Source: CAD feature listing. Evaluate the final solid. Frame: model axes, mm. A direction names the side the tool comes from. Give positions to 0.01 mm unless a question says otherwise; leave off trailing zeros. Order: outer loops, then holes, each group sorted by start corner. A loop starts at its lowest first (then second) coordinate and runs counter-clockwise, first axis right, second up.
```python
from build123d import *

# Parameters (mm, degrees)
SKETCH_1_R          = 31
EXTRUDE_1_DEPTH     = 1
SKETCH_2_R          = 28.27
EXTRUDE_2_DEPTH     = 11
SKETCH_3_R          = 31
EXTRUDE_3_DEPTH     = 1
SKETCH_4_R          = 19
EXTRUDE_4_DEPTH     = 8
SKETCH_5_R          = 4
CUT_EXTRUDE_1_DEPTH = 49.610698411


with BuildPart() as part:
    # Эскиз1 → Бобышка-Вытянуть1 (new body)
    with BuildSketch(Plane(origin=(0, 0, 0), x_dir=(1, 0, 0), z_dir=(0, 1, 0))):
        with Locations(Location((0, 0, 0), (0, 0, 270))):
            Circle(SKETCH_1_R)
    extrude(amount=EXTRUDE_1_DEPTH)

    # Эскиз2 → Бобышка-Вытянуть2 (add)
    with BuildSketch(Plane(origin=(0, 1, 0), x_dir=(1, 0, 0), z_dir=(0, 1, 0))):
        with Locations(Location((0, 0, 0), (0, 0, 270))):
            Circle(SKETCH_2_R)
    extrude(amount=EXTRUDE_2_DEPTH)

    # Эскиз3 → Бобышка-Вытянуть3 (add)
    with BuildSketch(Plane(origin=(0, 12, 0), x_dir=(1, 0, 0), z_dir=(0, 1, 0))):
        with Locations(Location((0, 0, 0), (0, 0, 270))):
            Circle(SKETCH_3_R)
    extrude(amount=EXTRUDE_3_DEPTH)

    # Эскиз4 → Бобышка-Вытянуть4 (add)
    with BuildSketch(Plane(origin=(0, 13, 0), x_dir=(1, 0, 0), z_dir=(0, 1, 0))):
        with Locations(Location((0, 0, 0), (0, 0, 270))):
            Circle(SKETCH_4_R)
    extrude(amount=EXTRUDE_4_DEPTH)

    # Эскиз5 → Вырез-Вытянуть1 (cut, through all)
    with BuildSketch(Plane(origin=(0, 21, 0), x_dir=(1, 0, 0), z_dir=(0, 1, 0))):
        with Locations(Location((0, 0, 0), (0, 0, 270))):
            Circle(SKETCH_5_R)
    extrude(amount=-CUT_EXTRUDE_1_DEPTH, mode=Mode.SUBTRACT)


solid = part.part
```
1) Reachability of faces 1 (the flat face through (-13.3, 13, -14.2)), 2 (the flat face through (-14, 1, 25)), 3 (the cylindrical face through (-3.905, 10.647, -0.867)) from +Z, -Z, +X, -X, +Y, -Y: full face, straight path, thin tool, end or side. Return the list, or none.
Report:
face 1: +Y
face 2: none
face 3: +Y, -Y
2) Pin query (flat end, axial travel): pin 1 (4 mm diameter, centred on x = 0, y = 7.5, fed in from -Z); pin 2 (4 mm diameter, centred on x = -3, y = 18.5, fed in from +Z); pin 3 (5 mm diameter, centred on y = 8.5, z = 20.5, fed in from -X). Return the tip coordinate at first contact, or that it passes through.
Report:
pin 1: stops at z = -28.27
pin 2: stops at z = 18.97
pin 3: stops at x = -21.8
3) Section query D-D, the plane x = -11. Return the cut outline in (y, z), and give its area (3 significant figures).
Report:
outline: (0, -28.98) - (1, -28.98) - (1, -26.04) - (12, -26.04) - (12, -28.98) - (13, -28.98) - (13, -15.49) - (21, -15.49) - (21, 15.49) - (13, 15.49) - (13, 28.98) - (12, 28.98) - (12, 26.04) - (1, 26.04) - (1, 28.98) - (0, 28.98) - close
area: 937 mm2
4) Section query C-C, the plane y = 1.75. Return the cut outline in (x, z), and give its area (3 significant figures).
Report:
outline: circle Ø56.54 at (0, 0); hole circle Ø8 at (0, 0)
area: 2,460 mm2
5) Draft query along Y for faces 4 (the flat face through (4.5, 21, -0.3)), 5 (the flat face through (-14, 12, 25)), 6 (the cylindrical face through (-11.56, 16.94, -15.08)), 7 (the flat face through (-6, 0, 0)). Return one class per face: +Y half, -Y half, draft (parallel to the pull), parting line (faces both ways), or undercut.
Report:
face 4: +Y half
face 5: undercut
face 6: draft
face 7: -Y half
6) Section query A-A, the plane x = 0. Return the cut outline in (y, z), and give its area (3 significant figures).
Report:
outline: (0, -31) - (1, -31) - (1, -28.27) - (12, -28.27) - (12, -31) - (13, -31) - (13, -19) - (21, -19) - (21, -4) - (0, -4) - close; (0, 4) - (21, 4) - (21, 19) - (13, 19) - (13, 31) - (12, 31) - (12, 28.27) - (1, 28.27) - (1, 31) - (0, 31) - close
area: 882 mm2
7) Material intervals for L1, parallel to X at y = 10.75, z = 0; L2, parallel to X at y = 14.75, z = 0; L3, parallel to Y at x = -16, z = 26, sorted ascending.
Report:
L1: x = -28.27 to -4, 4 to 28.27
L2: x = -19 to -4, 4 to 19
L3: y = 0 to 1, 12 to 13
8) Section query B-B, the plane z = 0. Return the cut outline in (x, y), and give its area (3 significant figures).
Report:
outline: (-31, 0) - (-4, 0) - (-4, 21) - (-19, 21) - (-19, 13) - (-31, 13) - (-31, 12) - (-28.27, 12) - (-28.27, 1) - (-31, 1) - close; (4, 0) - (31, 0) - (31, 1) - (28.27, 1) - (28.27, 12) - (31, 12) - (31, 13) - (19, 13) - (19, 21) - (4, 21) - close
area: 882 mm2
